Geometry check sheet. Reference: the model listing, model coordinates, mm. Round coordinates to 2 decimals unless told otherwise and drop trailing zeros. Write each loop counter-clockwise with the first axis right and the second up, starting at its lowest first coordinate (ties: lowest second). Pieces come first, ordered by that corner, then holes. Notation, with made-up numbers: (-2, 73.5) -> (52, 73.5) arc R23 cw to (52, 99.5) -> close; hole circle Ø7 at (-11, -32.5). An arc over 180 degrees is marked (long way). Use a Markdown table: item, result.
```python
from build123d import *

# Parameters (mm, degrees)
BOSS_EXTRUDE1_DEPTH = 10
BOSS_EXTRUDE2_START = 10
BOSS_EXTRUDE2_DEPTH = 17.5


with BuildPart() as part:
    # Sketch1 → Boss-Extrude1 (new body)
    with BuildSketch(Plane(origin=(0, 0, 0), x_dir=(1, 0, 0), z_dir=(0, 1, 0))):
        with BuildLine():
            Line((-8, -8.94427191), (-8, -9.604686356))
            ThreePointArc((-8, -9.604686356), (0, -12.5), (8, -9.604686356))
            Line((8, -9.604686356), (8, -8.94427191))
            ThreePointArc((8, -8.94427191), (0, -12), (-8, -8.94427191))
        make_face()
    extrude(amount=BOSS_EXTRUDE1_DEPTH)

    # Sketch1<3> → Boss-Extrude2 (add)
    with BuildSketch(Plane(origin=(0, 0, 0), x_dir=(1, 0, 0), z_dir=(0, 1, 0)).offset(BOSS_EXTRUDE2_START)):
        with BuildLine():
            Line((-12, 0), (-12.5, 0))
            ThreePointArc((-12.5, 0), (-11.319231423, -5.303300859), (-8, -9.604686356))
            Line((-8, -9.604686356), (-8, -8.94427191))
            ThreePointArc((-8, -8.94427191), (-10.95445115, -4.898979486), (-12, 0))
        make_face()
        with BuildLine():
            Line((-8, -8.94427191), (-8, -9.604686356))
            ThreePointArc((-8, -9.604686356), (0, -12.5), (8, -9.604686356))
            Line((8, -9.604686356), (8, -8.94427191))
            ThreePointArc((8, -8.94427191), (0, -12), (-8, -8.94427191))
        make_face()
        with BuildLine():
            Line((8, -8.94427191), (8, -9.604686356))
            ThreePointArc((8, -9.604686356), (11.319231423, -5.303300859), (12.5, 0))
            Line((12.5, 0), (12, 0))
            ThreePointArc((12, 0), (10.95445115, -4.898979486), (8, -8.94427191))
        make_face()
    extrude(amount=BOSS_EXTRUDE2_DEPTH)


solid = part.part
```
(1) Thickness scan on line 1 (X direction, y = 11.25, z = 10.75); line 2 (X direction, y = 11, z = 9); line 3 (Z direction, x = 0.25, y = 24.25). Record the ranges inside material, lowest first.
A:
| item | result |
|---|---|
| line 1 | x = -6.38 to -5.33, 5.33 to 6.38 |
| line 2 | x = -8.67 to -7.94, 7.94 to 8.67 |
| line 3 | z = 12 to 12.5 |
(2) Section check D-D on x = 4. Record the cut outline in (y, z).
A:
| item | result |
|---|---|
| outline | (0, 11.31) -> (27.5, 11.31) -> (27.5, 11.84) -> (0, 11.84) -> close |
(3) Gauge pin test, flat ends, axial feed: pin 1 Ø6 at (y, z) = (10, 7) entering from -X; pin 2 Ø0.5 at (y, z) = (5.5, 9.5) entering from -X; pin 3 Ø10 at (x, y) = (5.5, 4) entering from +Z. Record the tip position at first contact, or that the pin passes through.
A:
| item | result |
|---|---|
| pin 1 | stops at x = -11.84 |
| pin 2 | stops at x = -8 |
| pin 3 | stops at z = 12.49 |
(4) Section check B-B on y = 11.5. Record the cut outline in (x, z), plus the area to 3 significant figures.
A:
| item | result |
|---|---|
| outline | (-12.5, 0) -> (-12, 0) arc R12 cw to (12, 0) -> (12.5, 0) arc R12.5 ccw to start |
| area | 19.2 mm2 |
(5) Section check C-C on z = 4. Record the cut outline in (x, y).
A:
| item | result |
|---|---|
| outline | (-11.84, 10) -> (-11.31, 10) -> (-11.31, 27.5) -> (-11.84, 27.5) -> close; (11.31, 10) -> (11.84, 10) -> (11.84, 27.5) -> (11.31, 27.5) -> close |
(6) Section check A-A on z = 10.25. Record the cut outline in (x, y), plus the area to 3 significant figures.
A:
| item | result |
|---|---|
| outline | (-7.15, 0) -> (-6.24, 0) -> (-6.24, 27.5) -> (-7.15, 27.5) -> close; (6.24, 0) -> (7.15, 0) -> (7.15, 27.5) -> (6.24, 27.5) -> close |
| area | 50.3 mm2 |
